from build123d import *

# Parameters (mm, degrees)
BOSS_EXTRU_1_DEPTH = 15
CONG_1_R           = 10
SKETCH4_R          = 2
CUT_EXTRUDE3_DEPTH = 10
SKETCH5_R          = 2
CUT_EXTRUDE4_DEPTH = 10


with BuildPart() as part:
    # Esquisse1 → Boss.-Extru.1 (new, symmetric)
    with BuildSketch(Plane.XY):
        with BuildLine():
            Line((0, 2), (0, 27))
            Line((0, 27), (2, 27))
            Line((2, 27), (2, 2))
            Line((2, 2), (27, 2))
            Line((27, 2), (27, 0))
            Line((27, 0), (2, 0))
            ThreePointArc((2, 0), (0.585786438, 0.585786438), (0, 2))
        make_face()
    extrude(amount=BOSS_EXTRU_1_DEPTH, both=True)

    # Congé1
    cong_1_edges = [part.edges().sort_by_distance(p)[0] for p in [
        (27, 1, 15),
        (1, 27, 15),
        (27, 1, -15),
        (1, 27, -15),
    ]]
    fillet(cong_1_edges, radius=CONG_1_R)

    # Sketch4 → Cut-Extrude3 (cut)
    with BuildSketch(Plane(origin=(0, 2, 0), x_dir=(1, 0, 0), z_dir=(0, 1, 0))):
        with Locations(Location((7, 0, 0), (0, 0, 270))):
            Circle(SKETCH4_R)
        with Locations(Location((19, 0, 0), (0, 0, 270))):
            Circle(SKETCH4_R)
    extrude(amount=-CUT_EXTRUDE3_DEPTH, mode=Mode.SUBTRACT)

    # Sketch5 → Cut-Extrude4 (cut)
    with BuildSketch(Plane(origin=(2, 0, 0), x_dir=(0, 0, -1), z_dir=(1, 0, 0))):
        with Locations((-8, 19)):
            Circle(SKETCH5_R)
        with Locations((8, 19)):
            Circle(SKETCH5_R)
        with Locations((8, 7)):
            Circle(SKETCH5_R)
        with Locations((-8, 7)):
            Circle(SKETCH5_R)
    extrude(amount=-CUT_EXTRUDE4_DEPTH, mode=Mode.SUBTRACT)


solid = part.part
Can you work these out from the model? Positions are in its coordinate system, mm. A direction names the side the tool comes from. Give positions to 0.01 mm unless a question says otherwise; leave off trailing zeros. Loops run counter-clockwise (first coordinate to the right, second up) from the corner with the lowest first, then second, coordinate; pieces in that order, holes last. Notation, with made-up numbers: (57, -30.5) -> (101, -30.5) arc R25 ccw to (101, 8.5) -> close; hole circle Ø11 at (83.25, 77.5). An arc over 180 degrees is marked (long way). Return JSON: item names as keys, results as strings.
Q1. On a 3-axis mill with a long thin cutter (end or side, diameter ignored), from which of +Z, -Z, +X, -X, +Y, -Y can I reach the whole of each face in a straight line? I mean faces 4 (the face through (9, 1, 0)), 5 (the face through (2, 15, 0)). Say none if no direction works.
Checks:
{"face 4": "+Y, -Y", "face 5": "+Z, -Z, +X, +Y"}
Q2. I want a section at D-D, the plane x = 19. List the corners of the cut face in (y, z) for me.
Checks:
{"outline": "(0, -14.8) -> (2, -14.8) -> (2, -2) -> (0, -2) -> close; (0, 2) -> (2, 2) -> (2, 14.8) -> (0, 14.8) -> close"}
Q3. For pin 1 Ø6 at (y, z) = (5, 8) entering from -X; pin 2 Ø4 at (y, z) = (22.5, 4.5) entering from +X, each with a flat end and sliding along its axis, tell me the tip position at first contact or that it passes through.
Checks:
{"pin 1": "stops at x = 0", "pin 2": "stops at x = 2"}
Q4. I need wall thicknesses on probe 1 along Y at (x, z) = (0.8, -8); probe 2 along Y at (x, z) = (1.5, -8); probe 3 along X at (y, z) = (1.15, 0). Which ranges of each line are inside material? Lowest first, please.
Checks:
{"probe 1": "y = 0.4 to 5, 9 to 17, 21 to 26.54", "probe 2": "y = 0.06 to 5, 9 to 17, 21 to 26.54", "probe 3": "x = 0.19 to 5, 9 to 17, 21 to 27"}
Q5. I want a section at A-A, the plane y = 7. List the corners of the cut face in (x, z) for me, then the cut area to 3 significant figures.
Checks:
{"outline": "(0, -15) -> (2, -15) -> (2, -10) -> (0, -10) -> close; (0, -6) -> (2, -6) -> (2, 6) -> (0, 6) -> close; (0, 10) -> (2, 10) -> (2, 15) -> (0, 15) -> close", "area": "44.0 mm2"}
Q6. I want a section at B-B, the plane z = 0. List the corners of the cut face in (x, y) for me.
Checks:
{"outline": "(0, 2) arc R2 ccw to (2, 0) -> (5, 0) -> (5, 2) -> (2, 2) -> (2, 27) -> (0, 27) -> close; (9, 0) -> (17, 0) -> (17, 2) -> (9, 2) -> close; (21, 0) -> (27, 0) -> (27, 2) -> (21, 2) -> close"}
Q7. I want a section at C-C, the plane z = -13. List the corners of the cut face in (x, y) for me.
Checks:
{"outline": "(0, 2) arc R2 ccw to (2, 0) -> (23, 0) -> (23, 2) -> (2, 2) -> (2, 23) -> (0, 23) -> close"}
Q8. We'd pull the mould along Z, two halves only. Please class faces 1 (the face through (1, 21, -8)), 2 (the face through (23.99, 0.99, 12.15)), 3 (the face through (24.15, 0.99, -11.99)): released by +Z, released by -Z, zero draft, split by the parting line, or undercut.
Checks:
{"face 1": "undercut", "face 2": "released by +Z", "face 3": "released by -Z"}
